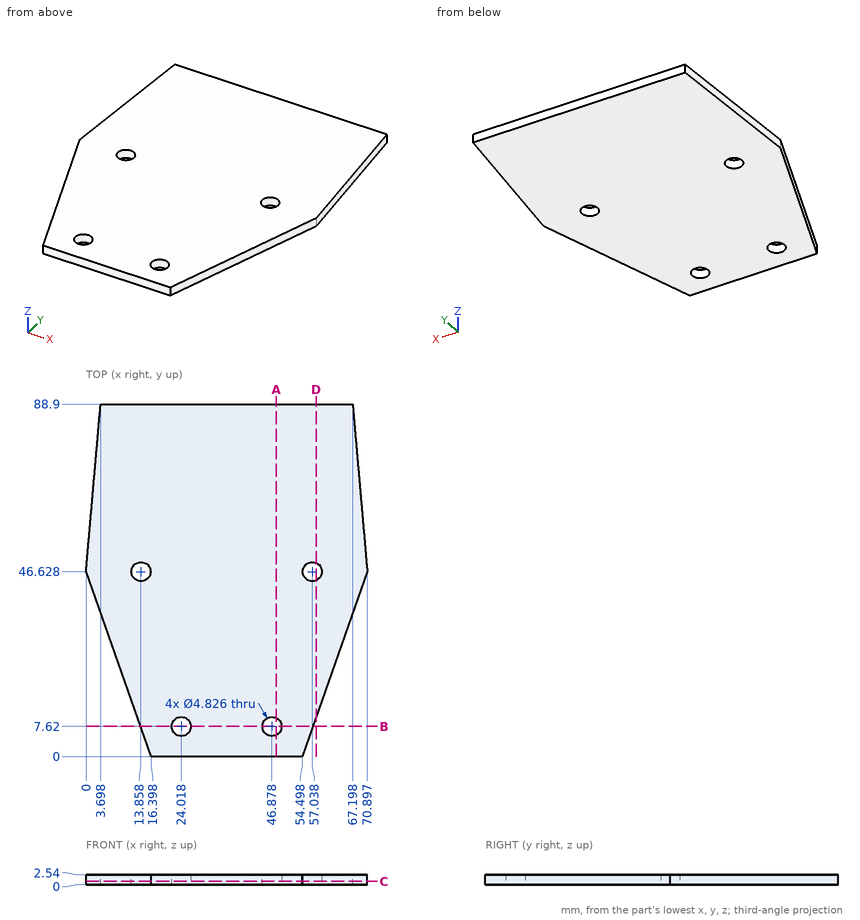
Input: dimensioned drawing with shaded views. Units: mm. Origin: part minimum x, y, z. Coordinates: 2 decimals unless noted, no trailing zeros. Loops run counter-clockwise (first coordinate to the right, second up) from the corner with the lowest first, then second, coordinate; pieces in that order, holes last. Notation, with made-up numbers: (14, 34) -> (40, 34) arc R17 cw to (40, 56) -> close; hole circle Ø8 at (52.25, -16.5). An arc over 180 degrees is marked (long way). Use a Markdown table: item, result. Add a question column.
(1) Section query D-D, the plane x = 58. Return loops of the section in (y, z) (1 decimal).
(2) Section query A-A, the plane x = 48. Return loops of the section in (y, z), plus the area to 3 significant figures.
(3) Line query: line 1 along Y through (x, z) = (46.5, 0.25); line 2 along Y through (x, z) = (23, 2); line 3 along X through (y, z) = (39.5, 0.9). Output: solid intervals per line, ascending.
(4) Section query B-B, the plane y = 7.62. Return loops of the section in (x, z) (1 decimal).
(5) Section query C-C, the plane z = 0.85. Return loops of the section in (x, y) (1 decimal).
Answer:
| question | item | result |
|---|---|---|
| 1 | outline | (10, 0) -> (44.4, 0) -> (44.4, 2.5) -> (10, 2.5) -> close; (48.8, 0) -> (88.9, 0) -> (88.9, 2.5) -> (48.8, 2.5) -> close |
| 2 | outline | (0, 0) -> (5.48, 0) -> (5.48, 2.54) -> (0, 2.54) -> close; (9.76, 0) -> (88.9, 0) -> (88.9, 2.54) -> (9.76, 2.54) -> close |
| 2 | area | 215 mm^2 |
| 3 | line 1 | y = 0 to 5.24, 10 to 88.9 |
| 3 | line 2 | y = 0 to 5.43, 9.81 to 88.9 |
| 3 | line 3 | x = 2.51 to 68.39 |
| 4 | outline | (13.7, 0) -> (21.6, 0) -> (21.6, 2.5) -> (13.7, 2.5) -> close; (26.4, 0) -> (44.5, 0) -> (44.5, 2.5) -> (26.4, 2.5) -> close; (49.3, 0) -> (57.2, 0) -> (57.2, 2.5) -> (49.3, 2.5) -> close |
| 5 | outline | (0, 46.6) -> (16.4, 0) -> (54.5, 0) -> (70.9, 46.6) -> (67.2, 88.9) -> (3.7, 88.9) -> close; hole circle Ø4.8 at (13.9, 46.6); hole circle Ø4.8 at (24, 7.6); hole circle Ø4.8 at (46.9, 7.6); hole circle Ø4.8 at (57, 46.6) |
